```python
from build123d import *

# Parameters (mm, degrees)
SKETCH_1_W      = 30
SKETCH_1_H      = 40
SKETCH_1_R      = 0.5
SKETCH_1_R_2    = 2
SKETCH_1_R_3    = 1.5
EXTRUDE_1_DEPTH = 1.5
SKETCH_2_R      = 9
SKETCH_2_R_2    = 4.5
EXTRUDE_2_DEPTH = 8
FILLET_1_R      = 1.8


with BuildPart() as part:
    # Эскиз1 → Вытянуть1 (new body)
    with BuildSketch(Plane.XY):
        Rectangle(SKETCH_1_W, SKETCH_1_H)
        with Locations((-12.7, -15.5)):
            Circle(SKETCH_1_R, mode=Mode.SUBTRACT)
        with Locations((-12.5, -5)):
            Circle(SKETCH_1_R, mode=Mode.SUBTRACT)
        with Locations((-7.62, -15.5)):
            Circle(SKETCH_1_R, mode=Mode.SUBTRACT)
        with Locations((-2.54, -15.5)):
            Circle(SKETCH_1_R, mode=Mode.SUBTRACT)
        with Locations((2.54, -15.5)):
            Circle(SKETCH_1_R, mode=Mode.SUBTRACT)
        with Locations((7.62, -15.5)):
            Circle(SKETCH_1_R, mode=Mode.SUBTRACT)
        with Locations((12.7, -15.5)):
            Circle(SKETCH_1_R, mode=Mode.SUBTRACT)
        with Locations((-7.5, -5)):
            Circle(SKETCH_1_R, mode=Mode.SUBTRACT)
        with Locations((-2.5, -5)):
            Circle(SKETCH_1_R, mode=Mode.SUBTRACT)
        with Locations((2.5, -5)):
            Circle(SKETCH_1_R, mode=Mode.SUBTRACT)
        with Locations((7.5, -5)):
            Circle(SKETCH_1_R, mode=Mode.SUBTRACT)
        with Locations((12.5, -5)):
            Circle(SKETCH_1_R, mode=Mode.SUBTRACT)
        with Locations((0, 10)):
            Circle(SKETCH_1_R_2, mode=Mode.SUBTRACT)
        with Locations((-12, 10)):
            Circle(SKETCH_1_R_3, mode=Mode.SUBTRACT)
        with Locations(Location((12, 10, 0), (0, 0, 180))):
            Circle(SKETCH_1_R_3, mode=Mode.SUBTRACT)
    extrude(amount=EXTRUDE_1_DEPTH)

    # Эскиз2 → Вытянуть2 (add)
    with BuildSketch(Plane.XY.offset(1.5)):
        with Locations(Location((0, 10, 0), (0, 0, 180))):
            Circle(SKETCH_2_R)
        with Locations((0, 10)):
            Circle(SKETCH_2_R_2, mode=Mode.SUBTRACT)
    extrude(amount=EXTRUDE_2_DEPTH)

    # Скругление1
    fillet_1_edges = [part.edges().sort_by_distance(p)[0] for p in [
        (9, 10, 9.5),
        (-4.5, 10, 9.5),
    ]]
    fillet(fillet_1_edges, radius=FILLET_1_R)


solid = part.part
```
The model under review builds one solid part; all positions refer to its coordinate system, in mm. A direction names the side the tool comes from. Round coordinates to 2 decimals unless told otherwise and drop trailing zeros. Loops run counter-clockwise (first coordinate to the right, second up) from the corner with the lowest first, then second, coordinate; pieces in that order, holes last. Notation, with made-up numbers: (55, 5) - (76, 5) arc R10 ccw to (76, 24) - close; hole circle Ø3 at (38, -29). An arc over 180 degrees is marked (long way). Use a Markdown table: item, result. Add a question column.
Q1. Add section A-A (y = -5). State the section outline as (x, z) points.
Q2. Machinability: for faces 4 (the face through (-15, 0, 1)), 5 (the face through (7.14, 15.48, 4.56)), which of the approach directions +Z, -Z, +X, -X, +Y, -Y give a long, thin tool a straight path to every point of the face, cutting with its end or side? Answer none if there is none.
Q3. Insertion check: pin 1 Ø2 at (y, z) = (5, 6.5) entering from +X; pin 2 Ø4 at (x, y) = (-12, 10) entering from +Z; pin 3 Ø4.5 at (x, y) = (2, 8.5) entering from +Z. Each pin has a flat end and moves straight along its axis. Give the tip position at first contact, or say it passes through.
Q4. For probe 1 along Y at (x, z) = (2.5, 1); probe 2 along Z at (x, y) = (9.25, -5); probe 3 along Y at (x, z) = (12.5, 0.5), list the stretches that pass through material, from the lowest coordinate up.
Q5. The part is to be moulded in two halves that separate along Y. For faces 1 (the face through (-13.1, -15.2, 0.7)), 2 (the face through (0, 20, 1)), 3 (the face through (0, -20, 1)), say which applies: pulls with the +Y half, pulls with the -Y half, needs draft (parallel to the pull), parting line crosses it, or undercut.
Q6. Add section B-B (x = 0). State the section outline as (y, z) points, plus the area to 3 significant figures.
Q7. Add section C-C (x = 9.5). State the section outline as (y, z) points, plus the area to 3 significant figures.
Worked answers:
| question | item | result |
|---|---|---|
| 1 | outline | (-15, 0) - (-13, 0) - (-13, 1.5) - (-15, 1.5) - close; (-12, 0) - (-8, 0) - (-8, 1.5) - (-12, 1.5) - close; (-7, 0) - (-3, 0) - (-3, 1.5) - (-7, 1.5) - close; (-2, 0) - (2, 0) - (2, 1.5) - (-2, 1.5) - close; (3, 0) - (7, 0) - (7, 1.5) - (3, 1.5) - close; (8, 0) - (12, 0) - (12, 1.5) - (8, 1.5) - close; (13, 0) - (15, 0) - (15, 1.5) - (13, 1.5) - close |
| 2 | face 4 | +Z, -Z, -X, +Y, -Y |
| 2 | face 5 | +Z |
| 3 | pin 1 | x = 8.06 |
| 3 | pin 2 | z = 1.5 |
| 3 | pin 3 | z = 8.62 |
| 4 | probe 1 | -20 to -16, -15 to -5.5, -4.5 to 20 |
| 4 | probe 2 | 0 to 1.5 |
| 4 | probe 3 | -20 to -15.96, -15.04 to -5.5, -4.5 to 8.59, 11.41 to 20 |
| 5 | face 1 | undercut |
| 5 | face 2 | pulls with the +Y half |
| 5 | face 3 | pulls with the -Y half |
| 6 | outline | (-20, 0) - (8, 0) - (8, 1.5) - (5.5, 1.5) - (5.5, 7.7) arc R1.8 ccw to (3.7, 9.5) - (2.8, 9.5) arc R1.8 ccw to (1, 7.7) - (1, 1.5) - (-20, 1.5) - close; (12, 0) - (20, 0) - (20, 1.5) - (19, 1.5) - (19, 7.7) arc R1.8 ccw to (17.2, 9.5) - (16.3, 9.5) arc R1.8 ccw to (14.5, 7.7) - (14.5, 1.5) - (12, 1.5) - close |
| 6 | area | 123 mm² |
| 7 | outline | (-20, 0) - (20, 0) - (20, 1.5) - (-20, 1.5) - close |
| 7 | area | 60.0 mm² |
